The model under review builds one solid part; all positions refer to its coordinate system, in mm. A direction names the side the tool comes from. Round coordinates to 2 decimals unless told otherwise and drop trailing zeros. Loops run counter-clockwise (first coordinate to the right, second up) from the corner with the lowest first, then second, coordinate; pieces in that order, holes last. Notation, with made-up numbers: M 57,27.25 L 69,27.25 A26 cw 69,42.25 Z; hole C 73,52.5 d3. An arc over 180 degrees is marked long. Use a Markdown table: item, result. Add a question column.
```python
from build123d import *

# Parameters (mm, degrees)
SKETCH1_R                                        = 50.8
BOSS_EXTRUDE1_DEPTH                              = 10.16
SKETCH2_R                                        = 5.15
CUT_EXTRUDE1_DEPTH                               = 11.16
CUT_EXTRUDE10_DEPTH                              = 1
CUT_EXTRUDE10_DEPTH_BACK                         = 11.16
CBORE_FOR_4_SOCKET_HEAD_CAP_SCREW1_AT_2_COUNT    = 2
CBORE_FOR_4_SOCKET_HEAD_CAP_SCREW1_AT_2_PITCH    = 65.991135768
CBORE_FOR_4_SOCKET_HEAD_CAP_SCREW1_AT_3_COUNT    = 2
CBORE_FOR_4_SOCKET_HEAD_CAP_SCREW1_AT_3_PITCH    = 76.2
CBORE_FOR_4_SOCKET_HEAD_CAP_SCREW1_AT_4_COUNT    = 2
CBORE_FOR_4_SOCKET_HEAD_CAP_SCREW1_AT_4_PITCH    = 38.1
CUT_EXTRUDE9_DEPTH                               = 11.16
F_4_40_TAPPED_HOLE1_D                            = 2.2606
CBORE_FOR_1_4_SOCKET_HEAD_CAP_SCREW1_D           = 6.7564
CBORE_FOR_1_4_SOCKET_HEAD_CAP_SCREW1_CBORE_D     = 11.1125
CBORE_FOR_1_4_SOCKET_HEAD_CAP_SCREW1_CBORE_DEPTH = 6.35
F_97_0_0059_DIAMETER_HOLE1_D                     = 1.27
F_4_40_TAPPED_HOLE2_D                            = 2.2606
F_4_40_TAPPED_HOLE2_DEPTH                        = 7.5946
F_4_40_TAPPED_HOLE2_CSINK_D                      = 4.1148
F_4_40_TAPPED_HOLE2_CSINK_ANGLE                  = 100
F_4_40_TAPPED_HOLE2_TIP                          = 0.679152758


with BuildPart() as part:
    # Sketch1 → Boss-Extrude1 (new body)
    with BuildSketch(Plane(origin=(0, 0, 0), x_dir=(1, 0, 0), z_dir=(0, 1, 0))):
        with Locations(Location((0, 0, 0), (0, 0, 270))):  # turned: the seam where the file's is
            Circle(SKETCH1_R)
    extrude(amount=BOSS_EXTRUDE1_DEPTH)

    # Sketch2 → Cut-Extrude1 (cut, through all)
    with BuildSketch(Plane(origin=(0, 10.16, 0), x_dir=(1, 0, 0), z_dir=(0, 1, 0))):
        with Locations(Location((0, 44.02963, 0), (0, 0, 270))):  # turned: the seam where the file's is
            Circle(SKETCH2_R)
        with Locations(Location((38.130778099, -22.014815, 0), (0, 0, 270))):  # turned: the seam where the file's is
            Circle(SKETCH2_R)
        with Locations(Location((-38.130778099, -22.014815, 0), (0, 0, 270))):  # turned: the seam where the file's is
            Circle(SKETCH2_R)
    extrude(amount=-CUT_EXTRUDE1_DEPTH, mode=Mode.SUBTRACT)

    # Sketch46 → Cut-Extrude10 (cut, two sides)
    with BuildSketch(Plane(origin=(0, 10.16, 0), x_dir=(1, 0, 0), z_dir=(0, 1, 0))) as cut_extrude10_sk:
        Polygon((47.092860393, 269.566399573), (47.092860393, 19.05), (47.092860393, -19.05), (47.092860393, -269.566399573), (548.12565954, -269.566399573), (548.12565954, 269.566399573), align=None)
    extrude(amount=CUT_EXTRUDE10_DEPTH, mode=Mode.SUBTRACT)
    extrude(cut_extrude10_sk.sketch, amount=-CUT_EXTRUDE10_DEPTH_BACK, mode=Mode.SUBTRACT)

    # Sketch38 → CBORE for #4 Socket Head Cap Screw1 (revolve, cut)
    with BuildSketch(Plane(origin=(19.05, 10.16, -32.995567884), x_dir=(0, 0, 1), z_dir=(1, 0, 0))):
        Polygon((0, 0), (0, 10.16), (1.63195, 10.16), (1.63195, 2.8448), (2.77876, 2.8448), (2.77876, 0.066070705), (2.8575, 0), align=None)
    cbore_for_4_socket_head_cap_screw1 = revolve(axis=Axis((19.05, 16.51, -32.995567884), (0, -1, 0)), mode=Mode.SUBTRACT)

    # CBORE for #4 Socket Head Cap Screw1 at 2: CBORE for #4 Socket Head Cap Screw1 ×2
    with Locations(*[(0, 0, i * CBORE_FOR_4_SOCKET_HEAD_CAP_SCREW1_AT_2_PITCH) for i in range(1, CBORE_FOR_4_SOCKET_HEAD_CAP_SCREW1_AT_2_COUNT)]):
        add(cbore_for_4_socket_head_cap_screw1, mode=Mode.SUBTRACT)

    # CBORE for #4 Socket Head Cap Screw1 at 3: CBORE for #4 Socket Head Cap Screw1 ×2
    with Locations(*[Vector(-0.5, 0, 0.866025404) * (i * CBORE_FOR_4_SOCKET_HEAD_CAP_SCREW1_AT_3_PITCH) for i in range(1, CBORE_FOR_4_SOCKET_HEAD_CAP_SCREW1_AT_3_COUNT)]):
        add(cbore_for_4_socket_head_cap_screw1, mode=Mode.SUBTRACT)

    # CBORE for #4 Socket Head Cap Screw1 at 4: CBORE for #4 Socket Head Cap Screw1 ×2
    with Locations(*[(-i * CBORE_FOR_4_SOCKET_HEAD_CAP_SCREW1_AT_4_PITCH, 0, 0) for i in range(1, CBORE_FOR_4_SOCKET_HEAD_CAP_SCREW1_AT_4_COUNT)]):
        add(cbore_for_4_socket_head_cap_screw1, mode=Mode.SUBTRACT)

    # Sketch39 → Cut-Extrude9 (cut, through all)
    with BuildSketch(Plane(origin=(0, 10.16, 0), x_dir=(1, 0, 0), z_dir=(0, 1, 0))):
        with BuildLine():
            Line((-39.37, 12.7), (-39.37, -12.7))
            ThreePointArc((-39.37, -12.7), (-38.626051224, -14.496051224), (-36.83, -15.24))
            Line((-36.83, -15.24), (-11.43, -15.24))
            ThreePointArc((-11.43, -15.24), (-9.633948776, -14.496051224), (-8.89, -12.7))
            Line((-8.89, -12.7), (-8.89, 12.7))
            ThreePointArc((-8.89, 12.7), (-9.633948776, 14.496051224), (-11.43, 15.24))
            Line((-11.43, 15.24), (-36.83, 15.24))
            ThreePointArc((-36.83, 15.24), (-38.626051224, 14.496051224), (-39.37, 12.7))
        make_face()
    extrude(amount=-CUT_EXTRUDE9_DEPTH, mode=Mode.SUBTRACT)

    # #4-40 Tapped Hole1 (through all)
    with Locations(Plane(origin=(0, 10.16, 0), x_dir=(1, 0, 0), z_dir=(0, 1, 0))):
        with Locations((7.62, 0), (-3.81, -6.599113577), (-3.81, 6.599113577)):
            Hole(F_4_40_TAPPED_HOLE1_D / 2)

    # CBORE for 1/4 Socket Head Cap Screw1 (through all)
    with Locations(Plane(origin=(0, 0, 0), x_dir=(-1, 0, 0), z_dir=(0, -1, 0))):
        with Locations((0, 0)):
            CounterBoreHole(CBORE_FOR_1_4_SOCKET_HEAD_CAP_SCREW1_D / 2, CBORE_FOR_1_4_SOCKET_HEAD_CAP_SCREW1_CBORE_D / 2, CBORE_FOR_1_4_SOCKET_HEAD_CAP_SCREW1_CBORE_DEPTH)

    # #97 (0.0059) Diameter Hole1 (through all)
    with Locations(Plane(origin=(0, 10.16, 0), x_dir=(1, 0, 0), z_dir=(0, 1, 0))):
        with Locations((40.132, 6.310189161), (40.132, -6.310189161)):
            Hole(F_97_0_0059_DIAMETER_HOLE1_D / 2)

    # #4-40 Tapped Hole2
    with Locations(Plane(origin=(47.092860393, 0, 0), x_dir=(0, 0, -1), z_dir=(1, 0, 0))):
        with Locations((-6.35, 7.62), (-6.35, 2.54), (6.35, 7.62), (6.35, 2.54)):
            CounterSinkHole(F_4_40_TAPPED_HOLE2_D / 2, F_4_40_TAPPED_HOLE2_CSINK_D / 2, depth=F_4_40_TAPPED_HOLE2_DEPTH, counter_sink_angle=F_4_40_TAPPED_HOLE2_CSINK_ANGLE)
            with Locations((0, 0, -(F_4_40_TAPPED_HOLE2_DEPTH + F_4_40_TAPPED_HOLE2_TIP / 2))):  # 118° drill point
                Cone(0, F_4_40_TAPPED_HOLE2_D / 2, F_4_40_TAPPED_HOLE2_TIP, mode=Mode.SUBTRACT)


solid = part.part
```
(1) Consider section B-B, the plane x = -19.05. Give the boundary of the cut face in (y, z).
(2) To check wall thickness, follow probe 1 along Y at (x, z) = (42.75, -6.35); probe 2 along X at (y, z) = (6, 4); probe 3 along Z at (x, y) = (18.5, 5.5). State the ranges of each line that lie inside material, in increasing order.
(3) Draft analysis for pull direction X (two halves, no side actions). For faces 4 (the face through (38.937, 7.428, -6.307)), 5 (the face through (-9.654, 5.151, 14.516)), 6 (the face through (10, 10.16, -1)), state which applies: released by +X, released by -X, zero draft, split by the parting line, or undercut.
(4) For faces 1 (the face through (18.215, 8.724, -30.345)), 2 (the face through (-9.614, 5.151, -14.476)), 3 (the face through (42.86, 8.57, -5.74)), list the 3-axis set-ups (+Z, -Z, +X, -X, +Y, -Y) from which the entire face can be reached by the end or side of a thin tool; tool diameter is ignored.
(5) Consider section D-D, the plane z = -27.5. Give the boundary of the cut face in (x, y).
(6) Insertion check: pin 1 Ø2 at (x, z) = (-19.05, 33) entering from +Y; pin 2 Ø4 at (x, y) = (0.5, 4.5) entering from +Z; pin 3 Ø5 at (x, y) = (-27, 5.5) entering from -Z; pin 4 Ø1.4 at (y, z) = (7.62, 6.35) entering from +X. Each pin has a flat end and moves straight along its axis. Give the tip position at first contact, or say it passes through.
(7) Consider section A-A, the plane x = 19.05. Give the boundary of the cut face in (y, z).
(8) Consider section C-C, the plane z = 33. Give the number of separate pieces and of enclosed holes in the cut face, then the cut area to 3 significant figures.
Found:
| question | item | result |
|---|---|---|
| 1 | outline | M 0,-47.09 L 10.16,-47.09 L 10.16,-35.85 L 10.09,-35.77 L 7.32,-35.77 L 7.32,-34.63 L 0,-34.63 Z; M 0,-31.36 L 7.32,-31.36 L 7.32,-30.22 L 10.09,-30.22 L 10.16,-30.14 L 10.16,-15.24 L 0,-15.24 Z; M 0,15.24 L 10.16,15.24 L 10.16,30.14 L 10.09,30.22 L 7.32,30.22 L 7.32,31.36 L 0,31.36 Z; M 0,34.63 L 7.32,34.63 L 7.32,35.77 L 10.09,35.77 L 10.16,35.85 L 10.16,47.09 L 0,47.09 Z |
| 2 | probe 1 | y = 0 to 1.41, 3.67 to 6.49, 8.75 to 10.16 |
| 2 | probe 2 | x = -50.64 to -39.37, -8.89 to -3.86, 3.86 to 47.09 |
| 2 | probe 3 | z = -47.31 to -34.53, -31.46 to 31.46, 34.53 to 47.31 |
| 3 | face 4 | released by +X |
| 3 | face 5 | undercut |
| 3 | face 6 | zero draft |
| 4 | face 1 | +Y |
| 4 | face 2 | +Y, -Y |
| 4 | face 3 | +X |
| 5 | outline | M -42.71,0 L 42.71,0 L 42.71,10.16 L -42.71,10.16 Z |
| 6 | pin 1 | passes through |
| 6 | pin 2 | stops at z = 50.8 |
| 6 | pin 3 | stops at z = -44.5 |
| 6 | pin 4 | stops at x = 39.24 |
| 7 | outline | M 0,-47.09 L 10.16,-47.09 L 10.16,-35.85 L 10.09,-35.77 L 7.32,-35.77 L 7.32,-34.63 L 0,-34.63 Z; M 0,-31.36 L 7.32,-31.36 L 7.32,-30.22 L 10.09,-30.22 L 10.16,-30.14 L 10.16,30.14 L 10.09,30.22 L 7.32,30.22 L 7.32,31.36 L 0,31.36 Z; M 0,34.63 L 7.32,34.63 L 7.32,35.77 L 10.09,35.77 L 10.16,35.85 L 10.16,47.09 L 0,47.09 Z |
| 8 | separate pieces | 3 |
| 8 | enclosed holes | 0 |
| 8 | area | 705 mm^2 |
